```python
from build123d import *

# Parameters (mm, degrees)
SKETCH1_R                                           = 6
BOSS_EXTRUDE1_DEPTH                                 = 8
CBORE_FOR_6_BINDING_HEAD_MACHINE_SCREW2_D           = 3.7973
CBORE_FOR_6_BINDING_HEAD_MACHINE_SCREW2_CBORE_D     = 7.9375
CBORE_FOR_6_BINDING_HEAD_MACHINE_SCREW2_CBORE_DEPTH = 2.2098
CHAMFER1_SIZE                                       = 1


with BuildPart() as part:
    # Sketch1 → Boss-Extrude1 (new body)
    with BuildSketch(Plane(origin=(0, 0, 0), x_dir=(1, 0, 0), z_dir=(0, 1, 0))):
        Circle(SKETCH1_R)
    extrude(amount=BOSS_EXTRUDE1_DEPTH)

    # CBORE for #6 Binding Head Machine Screw2 (through all)
    with Locations(Plane(origin=(0, 8, 0), x_dir=(1, 0, 0), z_dir=(0, 1, 0))):
        with Locations((0, 0)):
            CounterBoreHole(CBORE_FOR_6_BINDING_HEAD_MACHINE_SCREW2_D / 2, CBORE_FOR_6_BINDING_HEAD_MACHINE_SCREW2_CBORE_D / 2, CBORE_FOR_6_BINDING_HEAD_MACHINE_SCREW2_CBORE_DEPTH)

    # Chamfer1
    chamfer1_edges = [part.edges().sort_by_distance(p)[0] for p in [
        (-6, 0, 0),
    ]]
    chamfer(chamfer1_edges, length=CHAMFER1_SIZE)


solid = part.part
```
Part model, mm, in its own coordinate system. A direction names the side the tool comes from. Round coordinates to 2 decimals unless told otherwise and drop trailing zeros. Loops run counter-clockwise (first coordinate to the right, second up) from the corner with the lowest first, then second, coordinate; pieces in that order, holes last. Notation, with made-up numbers: (42, -8) -> (63, -8) arc R32 cw to (63, 20) -> close; hole circle Ø7 at (64, 86). An arc over 180 degrees is marked (long way). Use one line per item in the form item = value. Start each with the question number.
Item 1: Drop flat-ended pins along their axis: pin 1 Ø1.5 at (x, y) = (1, 3.5) entering from +Z; pin 2 Ø3 at (y, z) = (6.5, 4) entering from -X; pin 3 Ø7 at (x, z) = (0, 0) entering from +Y. Give the stop position or say it passes through.
Item 2: Tool access for faces 1 (the flat face through (2, 5.79, -1)), 2 (the flat face through (-0.1, 0, 2.2)): list every direction of +Z, -Z, +X, -X, +Y, -Y with a clear straight run to the whole face (end or side of a thin tool).
Item 3: Two-plate mould, pull along X, no slides. Class faces 3 (the cylindrical face through (-6, 4, 0)), 4 (the flat face through (1, 8, 4)), 5 (the cylindrical face through (-1.8, 2.9, -0.6)): released by +X, released by -X, zero draft, split by the parting line, or undercut.
Item 4: Band-saw the part on A-A (z = 0). List the corners of the cut face in (x, y), plus the area to 3 significant figures.
Item 5: Band-saw the part on D-D (y = 6.5). List the corners of the cut face in (x, z), plus the area to 3 significant figures.
Item 6: Band-saw the part on C-C (y = 5.5). List the corners of the cut face in (x, z).
Item 7: Drill centre lines: line 1 along Z through (x, y) = (0, 6.8); line 2 along Z through (x, y) = (0, 4.15); line 3 along Y through (x, z) = (1.5, -2.25). Where is each one in solid material? Low to high.
Item 8: Band-saw the part on B-B (x = 0). List the corners of the cut face in (y, z), plus the area to 3 significant figures.
Data:
q1.pin_1 = 5.99
q1.pin_2 = -5.45
q1.pin_3 = 5.79
q2.face_1 = +Y
q2.face_2 = +Z, -Z, +X, -X, -Y
q3.face_3 = split by the parting line
q3.face_4 = zero draft
q3.face_5 = undercut
q4.outline = (-6, 1) -> (-5, 0) -> (-1.9, 0) -> (-1.9, 5.79) -> (-3.97, 5.79) -> (-3.97, 8) -> (-6, 8) -> close; (1.9, 0) -> (5, 0) -> (6, 1) -> (6, 8) -> (3.97, 8) -> (3.97, 5.79) -> (1.9, 5.79) -> close
q4.area = 55.5 mm^2
q5.outline = circle Ø12 at (0, 0); hole circle Ø7.94 at (0, 0)
q5.area = 63.6 mm^2
q6.outline = circle Ø12 at (0, 0); hole circle Ø3.8 at (0, 0)
q7.line_1 = -6 to -3.97, 3.97 to 6
q7.line_2 = -6 to -1.9, 1.9 to 6
q7.line_3 = 0 to 5.79
q8.outline = (0, -5) -> (1, -6) -> (8, -6) -> (8, -3.97) -> (5.79, -3.97) -> (5.79, -1.9) -> (0, -1.9) -> close; (0, 1.9) -> (5.79, 1.9) -> (5.79, 3.97) -> (8, 3.97) -> (8, 6) -> (1, 6) -> (0, 5) -> close
q8.area = 55.5 mm^2
